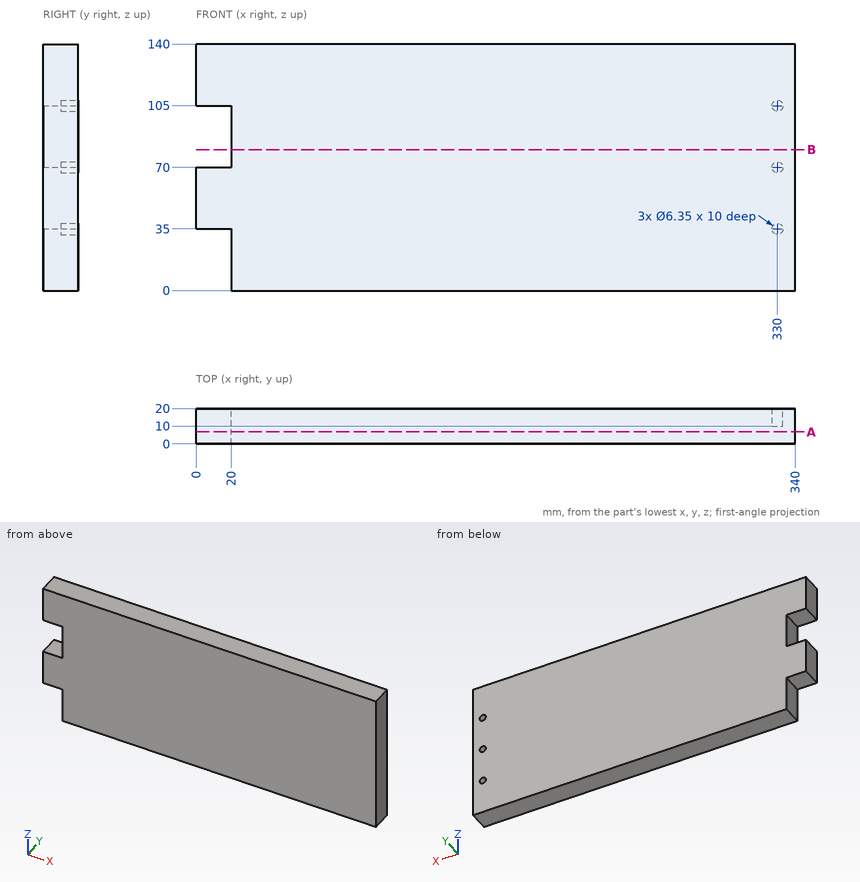
Here's the drawing with two shaded views (mm, measured from the low corner). I have some questions. Round coordinates to 2 decimals unless told otherwise and drop trailing zeros. Loops run counter-clockwise (first coordinate to the right, second up) from the corner with the lowest first, then second, coordinate; pieces in that order, holes last. Notation, with made-up numbers: (29.25, 77.25) - (79.25, 77.25) arc R24 ccw to (79.25, 112.25) - close; hole circle Ø1 at (-33.5, 21.5). An arc over 180 degrees is marked (long way). Use CSV: the item, a comma, the result in double quotes. Start each with the question number.
1) Please list where this line runs through material, in increasing order: probe 1 along X at (y, z) = (6, 9.5). Write a range as [from, to].
2) If we section it at B-B on z = 80: Write out the boundary of the cut face in (x, y).
3) For pin 1 Ø12 at (x, y) = (109, 7.5) entering from -Z; pin 2 Ø4 at (y, z) = (4, 28) entering from -X; pin 3 Ø5.5 at (x, z) = (330, 105) entering from +Y, each with a flat end and sliding along its axis, tell me the tip position at first contact or that it passes through.
4) If we section it at A-A on y = 6.75: Write out the boundary of the cut face in (x, z).
Geometry results:
1,probe 1,"x = [20, 340]"
2,outline,"(20, 0) - (340, 0) - (340, 20) - (20, 20) - close"
3,pin 1,"stops at z = 0"
3,pin 2,"stops at x = 20"
3,pin 3,"stops at y = 10"
4,outline,"(0, 35) - (20, 35) - (20, 0) - (340, 0) - (340, 140) - (0, 140) - (0, 105) - (20, 105) - (20, 70) - (0, 70) - close"
